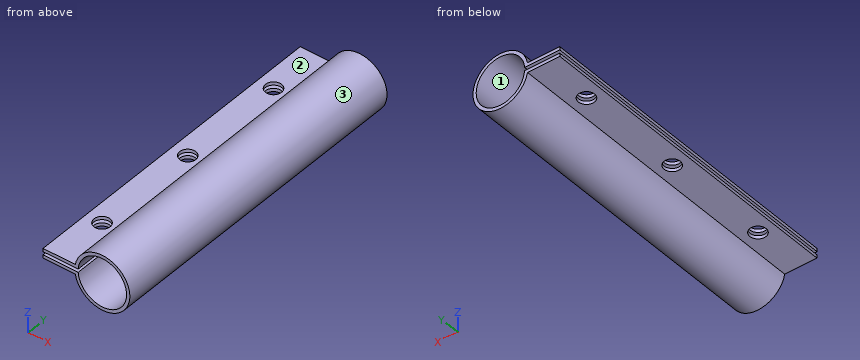
```python
from build123d import *

# Parameters (mm, degrees)
AUFSATZ_LINEAR_AUSTRAGEN1_DEPTH = 50
SKIZZE2_R                       = 1.25
SCHNITT_LINEAR_AUSTRAGEN1_DEPTH = 52.081630762


with BuildPart() as part:
    # Skizze1 → Aufsatz-Linear austragen1 (new body)
    with BuildSketch(Plane(origin=(0, 0, 0), x_dir=(1, 0, 0), z_dir=(0, 1, 0))):
        with BuildLine():
            Line((-4.183300133, 0.25), (-3.741657387, 0.25))
            ThreePointArc((-3.741657387, 0.25), (3.75, 0), (-3.741657387, -0.25))
            Line((-3.741657387, -0.25), (-4.183300133, -0.25))
            Line((-4.183300133, -0.25), (-9.183300133, -0.25))
            Line((-9.183300133, -0.25), (-9.183300133, -0.75))
            Line((-9.183300133, -0.75), (-4.183300133, -0.75))
            ThreePointArc((-4.183300133, -0.75), (4.25, 0), (-4.183300133, 0.75))
            Line((-4.183300133, 0.75), (-9.183300133, 0.75))
            Line((-9.183300133, 0.75), (-9.183300133, 0.25))
            Line((-9.183300133, 0.25), (-4.183300133, 0.25))
        make_face()
    extrude(amount=AUFSATZ_LINEAR_AUSTRAGEN1_DEPTH)

    # Skizze2 → Schnitt-Linear austragen1 (cut, through all)
    with BuildSketch(Plane.XY.offset(0.75)):
        with Locations((-6.683300133, 41.666666667)):
            Circle(SKIZZE2_R)
        with Locations((-6.683300133, 25)):
            Circle(SKIZZE2_R)
        with Locations((-6.683300133, 8.333333333)):
            Circle(SKIZZE2_R)
    extrude(amount=-SCHNITT_LINEAR_AUSTRAGEN1_DEPTH, mode=Mode.SUBTRACT)


solid = part.part
```
Geometry check sheet. Reference: the model listing, model coordinates, mm. Face numbers are marked on the shaded views. Give positions to 0.01 mm unless a question says otherwise; leave off trailing zeros. Loops run counter-clockwise (first coordinate to the right, second up) from the corner with the lowest first, then second, coordinate; pieces in that order, holes last. Notation, with made-up numbers: M 63.25,61 L 97.25,61 A21 ccw 97.25,85 Z; hole C 8,52.5 d6. An arc over 180 degrees is marked long. Write item = value, one per line. Start each with the question number.
1. Go/stop test with flat-tipped pins: P1, Ø4, axis at x = -6.68, y = 8.33, coming from the +Z side; P2, Ø1.5, axis at x = -7.5, y = 36.5, coming from the -Z side; P3, Ø2, axis at y = 44.5, z = -1.5, coming from the +X side. Record where each tip stops, or that it passes through.
2. Section check C-C, the plane z = -3.25. Enter the section's corners in (x, y).
3. Thickness scan on probe 1 along Z at (x, y) = (-5.25, 12); probe 2 along Z at (x, y) = (0.25, 14); probe 3 along X at (y, z) = (6.5, 1.25). Record the ranges inside material, lowest first.
4. Section check D-D, the plane y = 39. Enter the section's corners in (x, z).
5. Section check B-B, the plane y = 25. Enter the section's corners in (x, z), plus the area to 3 significant figures.
6. Section check A-A, the plane x = -5. Enter the section's corners in (y, z).
7. Draft check along X on the marked faces 1, 2 and 3. Enter one of: +X half, -X half, draft (parallel to the pull), parting line (faces both ways), or undercut.
Values follow:
q1.P1 = 0.75
q1.P2 = -0.75
q1.P3 = 4.22
q2.outline = M -2.74,0 L -1.87,0 L -1.87,50 L -2.74,50 Z; M 1.87,0 L 2.74,0 L 2.74,50 L 1.87,50 Z
q3.probe_1 = -0.75 to -0.25, 0.25 to 0.75
q3.probe_2 = -4.24 to -3.74, 3.74 to 4.24
q3.probe_3 = -4.06 to -3.54, 3.54 to 4.06
q4.outline = M -9.18,-0.75 L -4.18,-0.75 A4.25 ccw long -4.18,0.75 L -9.18,0.75 L -9.18,0.25 L -3.74,0.25 A3.75 cw long -3.74,-0.25 L -9.18,-0.25 Z
q5.outline = M -9.18,-0.75 L -7.93,-0.75 L -7.93,-0.25 L -9.18,-0.25 Z; M -9.18,0.25 L -7.93,0.25 L -7.93,0.75 L -9.18,0.75 Z; M -5.43,-0.75 L -4.18,-0.75 A4.25 ccw long -4.18,0.75 L -5.43,0.75 L -5.43,0.25 L -3.74,0.25 A3.75 cw long -3.74,-0.25 L -5.43,-0.25 Z
q5.area = 14.8 mm^2
q6.outline = M 0,-0.75 L 50,-0.75 L 50,-0.25 L 0,-0.25 Z; M 0,0.25 L 50,0.25 L 50,0.75 L 0,0.75 Z
q7.face_1 = undercut
q7.face_2 = draft
q7.face_3 = parting line
